Autodesk Inventor part; units mm, degrees
ref_plane "YZ Plane" through (0, 0, 0) normal (1, 0, 0) x (0, 1, 0)
ref_plane "XZ Plane" through (0, 0, 0) normal (0, 1, 0) x (-1, 0, 0)
ref_plane "XY Plane" through (0, 0, 0) normal (0, 0, 1) x (1, 0, 0)
sketch "Sketch1" plane through (0, 0, 0) normal (0, 0, 1) x (1, 0, 0)
  line L0 (0, 0) -> (0, 5)
  line L1 (18, 0) -> (18, 5)
  line L2 (0, 0) -> (18, 0)
  line L3 (0, 0) -> (18, 0)
  line L4 (18, 0) -> (18, 30)
  line L5 (18, 30) -> (0, 30)
  line L6 (0, 30) -> (0, 0)
  dimension "d0" = 30
extrude "Extrusion1" add sketch "Sketch1" along normal blind 5
fillet "Fillet1" radius 5 2 edges at (0, 30, 2.5) (18, 30, 2.5)
sketch "Sketch3" plane through (0, 0, 5) normal (0, 0, 1) x (1, 0, 0)
  circle A0 centre (9, 21) radius 2
  line L0 (0, 25) -> (0, 0)
  line L1 (13, 30) -> (5, 30)
  dimension "d11" = 9
  dimension "d12" = 9
  dimension "d13" = 4
hole "Hole2" at (9, 21, 5) direction (0, 0, -1) diameter 4 depth 20 tip angle 118
sketch "Sketch4" plane through (0, 0, 0) normal (0, -1, 0) x (1, 0, 0)
  circle A0 centre (3, 2.5) radius 1.5
  circle A1 centre (15, 2.5) radius 1.5
  line L0 (0, 0) -> (18, 0)
  line L1 (0, 0) -> (0, 5)
  dimension "d21" = 12
  dimension "d22" = 2.5
  dimension "d23" = 2.5
  dimension "d24" = 3
  dimension "d25" = 3
  dimension "d26" = 3
hole "Hole3" at (3, 0, 2.5) at (15, 0, 2.5) direction (0, 1, 0) diameter 2.459 depth 15 tip angle 118
equation "\"d14\" = d13"
properties part number "Z-Kettenhalter3"
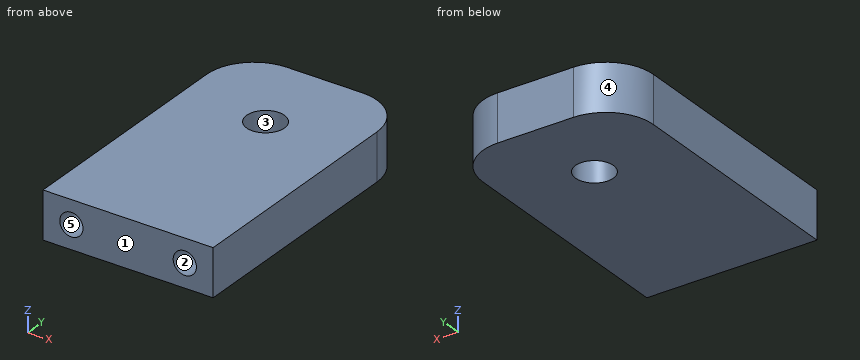
Can you work these out from the model? Positions are in its coordinate system, mm. Face numbers are marked on the shaded views. A direction names the side the tool comes from. Coordinates: 2 decimals unless noted, no trailing zeros. Loops run counter-clockwise (first coordinate to the right, second up) from the corner with the lowest first, then second, coordinate; pieces in that order, holes last. Notation, with made-up numbers: (-26.5, 89) -> (20.5, 89) arc R7 cw to (20.5, 95) -> close; hole circle Ø10 at (-0.75, 30.25). An arc over 180 degrees is marked (long way). Answer as a JSON object with one key per item and string values.
1) For P1, Ø3, axis at x = 9, y = 21, coming from the +Z side; P2, Ø1.5, axis at x = 4, y = 15.5, coming from the -Z side; P3, Ø1.5, axis at x = 3, z = 2.5, coming from the +Y side, each with a flat end and sliding along its axis, tell me the tip position at first contact or that it passes through.
Results:
{"P1": "passes through", "P2": "stops at z = 0", "P3": "stops at y = 29.84"}
2) Imagine slicing it at A-A (x = 9). Please give me the cut outline in (y, z).
Results:
{"outline": "(0, 0) -> (19, 0) -> (19, 5) -> (0, 5) -> close; (23, 0) -> (30, 0) -> (30, 5) -> (23, 5) -> close"}
3) If I drill on line 1 (X direction, y = 10.5, z = 2.5); line 2 (Z direction, x = 3, y = 5); line 3 (Y direction, x = 9, z = 2.25), over which ranges is the centre line in solid material (lowest first)?
Results:
{"line 1": "x = 0 to 1.77, 4.23 to 13.77, 16.23 to 18", "line 2": "z = 0 to 1.27, 3.73 to 5", "line 3": "y = 0 to 19, 23 to 30"}
4) Imagine slicing it at B-B (y = 20.5). Please give me the cut outline in (x, z), then the cut area to 3 significant figures.
Results:
{"outline": "(0, 0) -> (7.06, 0) -> (7.06, 5) -> (0, 5) -> close; (10.94, 0) -> (18, 0) -> (18, 5) -> (10.94, 5) -> close", "area": "70.6 mm^2"}
5) Thinking about a two-plate mould opening in Y: for the marked faces 3, 4 and 5, which applies, pulls with the +Y half, pulls with the -Y half, needs draft (parallel to the pull), parting line crosses it, or undercut?
Results:
{"face 3": "undercut", "face 4": "pulls with the +Y half", "face 5": "needs draft"}
6) For the marked faces 1 and 2, which set-ups out of +Z, -Z, +X, -X, +Y, -Y let a thin tool reach every point of the face, with its end or its side?
Results:
{"face 1": "+Z, -Z, +X, -X, -Y", "face 2": "-Y"}
7) Imagine slicing it at D-D (y = 28.25). Please give me the cut outline in (x, z).
Results:
{"outline": "(1.2, 0) -> (16.8, 0) -> (16.8, 5) -> (1.2, 5) -> close"}
8) Imagine slicing it at C-C (y = 11.5). Please give me the cut outline in (x, z), then the cut area to 3 significant figures.
Results:
{"outline": "(0, 0) -> (18, 0) -> (18, 5) -> (0, 5) -> close; hole circle Ø2.46 at (3, 2.5); hole circle Ø2.46 at (15, 2.5)", "area": "80.5 mm^2"}
